Design review of the part built by this model. Coordinates are the model's own, in mm. A direction names the side the tool comes from. Give positions to 0.01 mm unless a question says otherwise; leave off trailing zeros. Loops run counter-clockwise (first coordinate to the right, second up) from the corner with the lowest first, then second, coordinate; pieces in that order, holes last. Notation, with made-up numbers: (-13, -19.75) -> (1, -19.75) arc R24 ccw to (1, -4.75) -> close; hole circle Ø11 at (-21.5, -29.75). An arc over 180 degrees is marked (long way). Use CSV: the item, a comma, the result in double quotes. Start each with the question number.
Item 1: For faces 1 (the face through (-3, 6.5, 2)), 2 (the face through (2.15, 3.67, 1.74)), 3 (the face through (-9.914, 4, 2)), 4 (the face through (4.24, 6.18, 1.76)), 5 (the face through (-5, 1.5, 2)), list the 3-axis set-ups (+Z, -Z, +X, -X, +Y, -Y) from which the entire face can be reached by the end or side of a thin tool; tool diameter is ignored.
Item 2: We need section D-D (z = 0.5). State the section outline as (x, y) points.
Item 3: Wall thickness on line 1 along Y through (x, z) = (-2.25, 1.7); line 2 along Z through (x, y) = (-7.25, 6.6); line 3 along X through (y, z) = (1.9, 2.5): over which ranges is each line inside the solid? List them lowest first. Write a range as from..to.
Item 4: We need section A-A (z = 1.8). State the section outline as (x, y) points.
Item 5: We need section C-C (z = 2.8). State the section outline as (x, y) points.
Item 6: We need section B-B (x = -6.5). State the section outline as (y, z) points, plus the area to 3 significant figures.
Item 7: Clearance check with a flat-ended pin moving along its axis: pin 1 (1.6 mm diameter, centred on y = 3, z = 2, fed in from -X). State where the tip first meets the part, or that it passes through.
from build123d import *

# Parameters (mm, degrees)
BOSS_EXTRUDE1_DEPTH = 1
BOSS_EXTRUDE2_DEPTH = 2
FILLET1_R           = 0.5
FILLET2_R           = 0.5


with BuildPart() as part:
    # Sketch1 → Boss-Extrude1 (new body)
    with BuildSketch(Plane.XY):
        Polygon((0.185786438, 7), (6.185786438, 7), (0.185786438, 1), (-10.414213562, 1), (-10.414213562, 7), align=None)
    extrude(amount=BOSS_EXTRUDE1_DEPTH)

    # Sketch3 → Boss-Extrude2 (add)
    with BuildSketch(Plane.XY.offset(1)):
        Polygon((-0.621320344, 6.5), (4.978679656, 6.5), (-0.021320344, 1.5), (-9.914213562, 1.5), (-9.914213562, 6.5), align=None)
    extrude(amount=BOSS_EXTRUDE2_DEPTH)

    # Fillet1
    fillet1_edges = [part.edges().sort_by_distance(p)[0] for p in [
        (-9.914213562, 6.5, 2),
        (-9.914213562, 1.5, 2),
        (-0.021320344, 1.5, 2),
        (4.978679656, 6.5, 2),
    ]]
    fillet(fillet1_edges, radius=FILLET1_R)

    # Fillet2
    fillet2_edges = [part.edges().sort_by_distance(p)[0] for p in [
        (-2.821320344, 6.5, 3),
        (2.125126266, 3.646446609, 3),
        (-9.914213562, 4, 3),
        (-4.821320344, 1.5, 3),
        (-0.037085409, 1.538060234, 3),
        (-9.767766953, 1.646446609, 3),
        (-9.767766953, 6.353553391, 3),
        (4.233512642, 6.191341716, 3),
    ]]
    fillet(fillet2_edges, radius=FILLET2_R)


solid = part.part
Results found:
1,face 1,"+Z, +X, -X, +Y"
1,face 2,"+Z, +X, -Y"
1,face 3,"+Z, -X, +Y, -Y"
1,face 4,"+Z, +X"
1,face 5,"+Z, +X, -X, -Y"
2,outline,"(-10.41, 1) -> (0.19, 1) -> (6.19, 7) -> (-10.41, 7) -> close"
3,line 1,"1.5..6.5"
3,line 2,"0..1"
3,line 3,"-9.9..0.38"
4,outline,"(-9.91, 2) arc R0.5 ccw to (-9.41, 1.5) -> (-0.23, 1.5) arc R0.5 ccw to (0.13, 1.65) -> (4.13, 5.65) arc R0.5 ccw to (3.77, 6.5) -> (-9.41, 6.5) arc R0.5 ccw to (-9.91, 6) -> close"
5,outline,"(-9.81, 2) arc R0.4 ccw to (-9.41, 1.6) -> (-0.23, 1.6) arc R0.4 ccw to (0.05, 1.72) -> (4.05, 5.72) arc R0.4 ccw to (3.77, 6.4) -> (-9.41, 6.4) arc R0.4 ccw to (-9.81, 6) -> close"
6,outline,"(1, 0) -> (7, 0) -> (7, 1) -> (6.5, 1) -> (6.5, 2.5) arc R0.5 ccw to (6, 3) -> (2, 3) arc R0.5 ccw to (1.5, 2.5) -> (1.5, 1) -> (1, 1) -> close"
6,area,"15.9 mm²"
7,pin 1,"x = -9.91"
